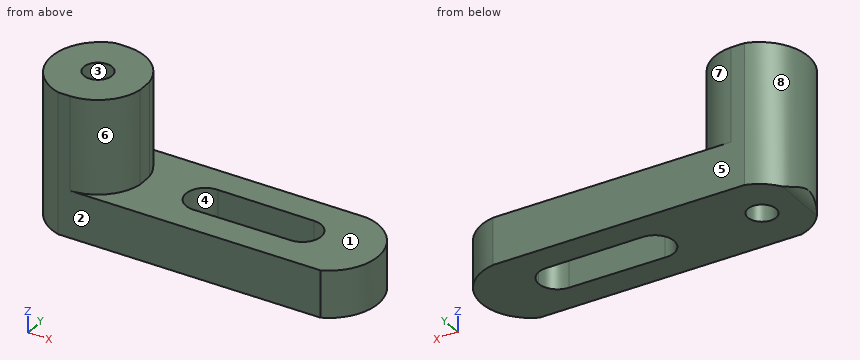
from build123d import *

# Parameters (mm, degrees)
F1_DEPTH  = 25.4
F3_DEPTH  = 25.4
F5_DEPTH  = 25.4
F7_DEPTH  = 25.4
F9_DEPTH  = 50.8
F13_DEPTH = 25.4
F14_R     = 3.8000451494
F15_DEPTH = 76.2
F17_DEPTH = 25.4


# Not quite as in the source:
# - the program builds the solid bodies; features that only make, move or delete a surface that nothing else refers to are left out


with BuildPart() as f1:
    # F0 (on Front) → F1 (new body)
    with BuildSketch(Plane.XZ):
        Polygon((-25.4, 38.1), (-25.4, 0), (63.5, 0), (63.5, 12.7), (0, 12.7), (0, 38.1), align=None)
    extrude(amount=F1_DEPTH)

    # F2 (on face) → F3 (cut)
    with BuildSketch(Plane.XZ.offset(25.4)):
        with BuildLine():
            ThreePointArc((-22.676864444, 0), (-24.571583371, 1.2835083224), (-25.4, 3.4168342035))
            Line((-25.4, 3.4168342035), (-25.4, 0))
            Line((-25.4, 0), (-22.676864444, 0))
        make_face()
    extrude(amount=-F3_DEPTH, mode=Mode.SUBTRACT)

    # F4 (on face) → F5 (cut)
    with BuildSketch(Plane.XY.offset(12.7)):
        with BuildLine():
            ThreePointArc((51.9632771611, 0), (63.0542215265, -11.5438688547), (55.0368912518, -25.4))
            Line((55.0368912518, -25.4), (63.5, -25.4))
            Line((63.5, -25.4), (63.5, 0))
            Line((63.5, 0), (51.9632771611, 0))
        make_face()
    extrude(amount=-F5_DEPTH, mode=Mode.SUBTRACT)

    # F6 (on face) → F7 (cut)
    with BuildSketch(Plane.XY.offset(38.1)):
        with BuildLine():
            ThreePointArc((-15.4641177505, -25.4), (-25.0669029781, -12.7718994312), (-15.6562179327, 0))
            Line((-15.6562179327, 0), (-25.4, 0))
            Line((-25.4, 0), (-25.4, -25.4))
            Line((-25.4, -25.4), (-15.4641177505, -25.4))
        make_face()
    extrude(amount=-F7_DEPTH, mode=Mode.SUBTRACT)

    # F8 (on face) → F9 (cut)
    with BuildSketch(Plane.XY.offset(12.7)):
        with BuildLine():
            Line((-25.4, 0), (-25.4, -25.4))
            Line((-25.4, -25.4), (-15.4641177505, -25.4))
            ThreePointArc((-15.4641177505, -25.4), (-25.0669029781, -12.7718994312), (-15.6562179327, 0))
            Line((-15.6562179327, 0), (-25.4, 0))
        make_face()
    extrude(amount=-F9_DEPTH, mode=Mode.SUBTRACT)

    # F12 (on face) → F13 (cut)
    with BuildSketch(Plane.XY.offset(38.1)):
        with BuildLine():
            ThreePointArc((-12.0063023642, 0), (-4.1167210002, -3.1788126596), (0, -10.6221286028))
            Line((0, -10.6221286028), (0, 0))
            Line((0, 0), (-12.0063023642, 0))
        make_face()
        with BuildLine():
            ThreePointArc((0, -14.7690480964), (-4.2265465157, -22.308409709), (-12.2979614132, -25.4))
            Line((-12.2979614132, -25.4), (0, -25.4))
            Line((0, -25.4), (0, -14.7690480964))
        make_face()
    extrude(amount=-F13_DEPTH, mode=Mode.SUBTRACT)

    # F14 (on face) → F15 (cut)
    with BuildSketch(Plane.XY.offset(38.1)):
        with Locations((-12.53633365, -12.6955883496)):
            Circle(F14_R)
    extrude(amount=-F15_DEPTH, mode=Mode.SUBTRACT)

    # F16 (on face) → F17 (cut)
    with BuildSketch(Plane.XY.offset(12.7)):
        with BuildLine():
            ThreePointArc((16.6168020143, -17.7693230367), (20.0435798879, -16.1217506564), (21.4334555491, -12.5826057047))
            ThreePointArc((21.4334555491, -12.5826057047), (19.9746784977, -8.9706846186), (16.4166737264, -7.3849335457))
            ThreePointArc((16.4166737264, -7.3849335457), (11.0325544335, -12.6828196506), (16.6168020143, -17.7693230367))
        make_face()
        with BuildLine():
            ThreePointArc((47.4116187176, -12.5826057047), (45.9414348271, -9.0192691511), (42.3863259992, -7.5292995919))
            ThreePointArc((42.3863259992, -7.5292995919), (37.304850424, -12.5816406618), (42.3843959412, -17.6359221781))
            ThreePointArc((42.3843959412, -17.6359221781), (45.9407542727, -16.1466264756), (47.4116187176, -12.5826057047))
        make_face()
        with BuildLine():
            ThreePointArc((16.4166737264, -7.3849335457), (19.9746784977, -8.9706846186), (21.4334555491, -12.5826057047))
            ThreePointArc((21.4334555491, -12.5826057047), (20.0435798879, -16.1217506564), (16.6168020143, -17.7693230367))
            Line((16.6168020143, -17.7693230367), (42.3843959412, -17.6359221781))
            ThreePointArc((42.3843959412, -17.6359221781), (37.304850424, -12.5816406618), (42.3863259992, -7.5292995919))
            Line((42.3863259992, -7.5292995919), (16.4166737264, -7.3849335457))
        make_face()
    extrude(amount=-F17_DEPTH, mode=Mode.SUBTRACT)


solid = f1.part
Read the model definition and answer for the solid it produces. Units are mm, in the model's axes. Face numbers are marked on the shaded views. A direction names the side the tool comes from. Coordinates: 2 decimals unless noted, no trailing zeros. Loops run counter-clockwise (first coordinate to the right, second up) from the corner with the lowest first, then second, coordinate; pieces in that order, holes last.
Q1. Consider probe 1 along Y at (x, z) = (18.5, 4); probe 2 along Y at (x, z) = (42.5, 3.5); probe 3 along Z at (x, y) = (31, -3.5). Determine where each line is inside the solid, lowest interval first.
Q2. The part is cut by section A-A on x = 22. Write down the section's boundary in (y, z), and give its area (3 significant figures).
Q3. Each of these flat-tipped pins is pushed along its axis until it touches: pin 1 Ø1 at (x, y) = (24.5, -16) entering from +Z; pin 2 Ø12.5 at (x, y) = (12, -9.5) entering from +Z; pin 3 Ø3 at (y, z) = (-22, 7.5) entering from -X; pin 4 Ø2 at (y, z) = (-12.5, 28) entering from +X. Where does it stop, or does it pass through?
Q4. The part is cut by section D-D on x = -3. Write down the section's boundary in (y, z).
Q5. The mould has two halves that part along Y. Classify the marked faces 1, 2 and 3: +Y half, -Y half, draft (parallel to the pull), parting line (faces both ways), or undercut.
Q6. Which of the six approach directions +Z, -Z, +X, -X, +Y, -Y give full straight-line access (tool end or side, diameter ignored) to the marked faces 4, 5, 6, 7 and 8?
Q7. The part is cut by section B-B on z = 32. Write down the section's boundary in (x, y), and give its area (3 significant figures).
Q8. The part is cut by section C-C on y = -21.5. Write down the section's boundary in (x, z).
Results below:
1. probe 1: y = -25.4 to -17.76, -7.4 to 0
1. probe 2: y = -25.4 to -17.63, -7.53 to 0
1. probe 3: z = 0 to 12.7
2. outline: (-25.4, 0) - (-17.74, 0) - (-17.74, 12.7) - (-25.4, 12.7) - close; (-7.42, 0) - (0, 0) - (0, 12.7) - (-7.42, 12.7) - close
2. area: 191 mm2
3. pin 1: passes through
3. pin 2: stops at z = 12.7
3. pin 3: stops at x = -22.5
3. pin 4: stops at x = 0
4. outline: (-25.4, 0) - (0, 0) - (0, 12.7) - (-4.3, 12.7) - (-4.3, 38.1) - (-21.09, 38.1) - (-21.09, 12.7) - (-25.4, 12.7) - close
5. face 1: draft
5. face 2: -Y half
5. face 3: undercut
6. face 4: +Z, -Z
6. face 5: +Z, -Z, +X, -X, +Y
6. face 6: +Z, +X, -Y
6. face 7: +Z, +X, +Y
6. face 8: +Z, -Z, -X
7. outline: (-15.66, 0) arc R13.24 ccw to (-15.46, -25.4) - (-12.3, -25.4) arc R12.71 ccw to (0, -14.77) - (0, -10.62) arc R12.71 ccw to (-12.01, 0) - close; hole circle Ø7.6 at (-12.54, -12.7)
7. area: 462 mm2
8. outline: (-21.69, 0) - (60.2, 0) - (60.2, 12.7) - (-3.37, 12.7) - (-3.37, 38.1) - (-21.69, 38.1) - close
